Part print with two shaded views. Sizes in mm from the minimum x, y, z corner. Round coordinates to 2 decimals unless told otherwise and drop trailing zeros. Loops run counter-clockwise (first coordinate to the right, second up) from the corner with the lowest first, then second, coordinate; pieces in that order, holes last. Notation, with made-up numbers: (77.25, 20) - (84.25, 20) arc R16 cw to (84.25, 51) - close; hole circle Ø8 at (-35, 37.25). An arc over 180 degrees is marked (long way). Use a Markdown table: item, result.
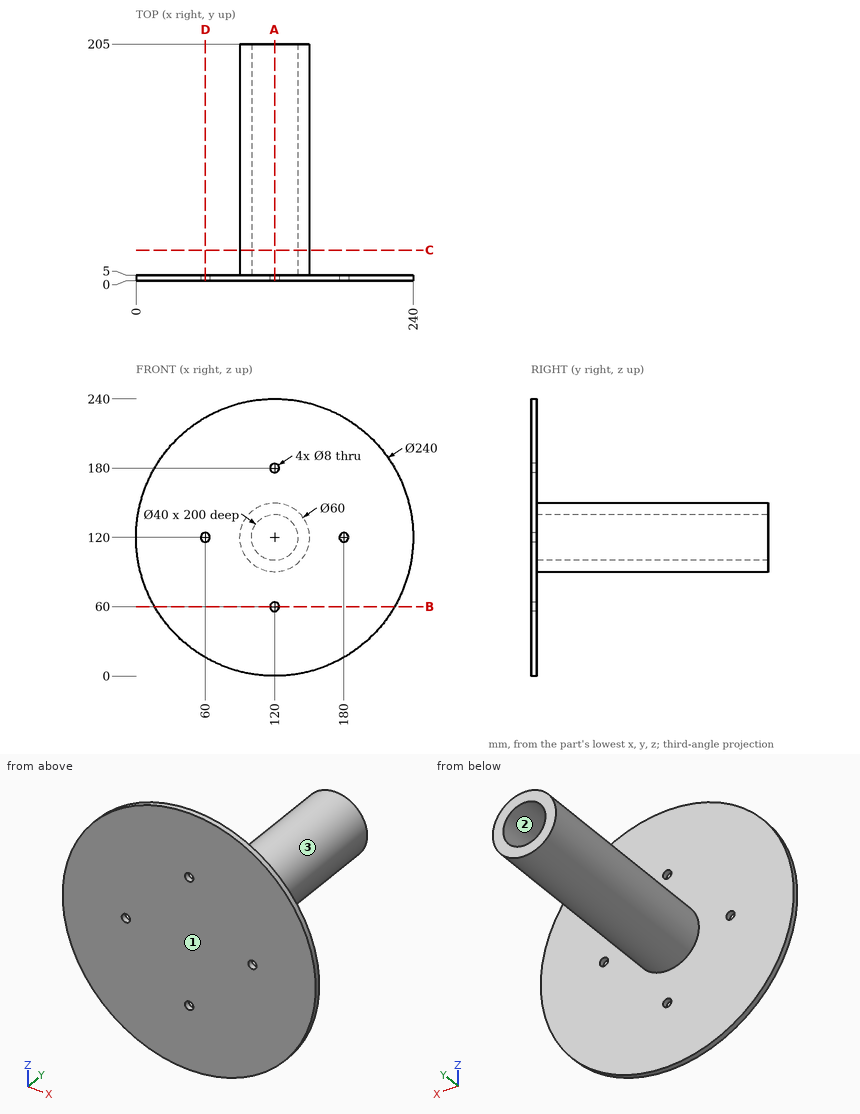
Q1. Cut at A-A, the plane x = 120. List the corners of the cut face in (y, z), plus the area to 3 significant figures.
Results found:
| item | result |
|---|---|
| outline | (0, 0) - (5, 0) - (5, 56) - (0, 56) - close; (0, 64) - (5, 64) - (5, 90) - (205, 90) - (205, 100) - (5, 100) - (5, 140) - (205, 140) - (205, 150) - (5, 150) - (5, 176) - (0, 176) - close; (0, 184) - (5, 184) - (5, 240) - (0, 240) - close |
| area | 5,120 mm2 |
Q2. Cut at C-C, the plane y = 26.5. List the corners of the cut face in (x, z).
Results found:
| item | result |
|---|---|
| outline | circle Ø60 at (120, 120); hole circle Ø40 at (120, 120) |
Q3. Cut at B-B, the plane z = 60. List the corners of the cut face in (x, y), plus the area to 3 significant figures.
Results found:
| item | result |
|---|---|
| outline | (16.08, 0) - (116, 0) - (116, 5) - (16.08, 5) - close; (124, 0) - (223.92, 0) - (223.92, 5) - (124, 5) - close |
| area | 999 mm2 |
Q4. Pull direction Z, two halves, no side cores. Call the marked faces 1, 2 and 3: pulls with the +Z half, pulls with the -Z half, needs draft (parallel to the pull), parting line crosses it, or undercut.
Results found:
| item | result |
|---|---|
| face 1 | needs draft |
| face 2 | undercut |
| face 3 | parting line crosses it |
Q5. Cut at D-D, the plane x = 60. List the corners of the cut face in (y, z), plus the area to 3 significant figures.
Results found:
| item | result |
|---|---|
| outline | (0, 16.08) - (5, 16.08) - (5, 116) - (0, 116) - close; (0, 124) - (5, 124) - (5, 223.92) - (0, 223.92) - close |
| area | 999 mm2 |
Q6. Drop flat-ended pins along their axis: pin 1 (8 mm diameter, centred on x = 128, y = 152.5, fed in from +Z); pin 2 (6 mm diameter, centred on x = 73, z = 122.5, fed in from +Y); pin 3 (12 mm diameter, centred on x = 139.5, y = 180.5, fed in from +Z). Give the stop position or say it passes through.
Results found:
| item | result |
|---|---|
| pin 1 | stops at z = 149.73 |
| pin 2 | stops at y = 5 |
| pin 3 | stops at z = 146.79 |
Q7. Probe line 1 (X direction, y = 3.3, z = 120); line 2 (Z direction, x = 121, y = 76); line 3 (X direction, y = 142.5, z = 120). List the from-to ranges inside material, lowest first.
Results found:
| item | result |
|---|---|
| line 1 | x = 0 to 56, 64 to 176, 184 to 240 |
| line 2 | z = 90.02 to 100.03, 139.97 to 149.98 |
| line 3 | x = 90 to 100, 140 to 150 |
